Read the model definition and answer for the solid it produces. Units are mm, in the model's axes. A direction names the side the tool comes from. Give positions to 0.01 mm unless a question says otherwise; leave off trailing zeros. Write each loop counter-clockwise with the first axis right and the second up, starting at its lowest first coordinate (ties: lowest second). Pieces come first, ordered by that corner, then holes.
```python
from build123d import *

# Parameters (mm, degrees)
F0_W     = 7.8
F0_H     = 7.8
F1_DEPTH = 1
F2_SIZE2 = 0.5
F2_SIZE  = 7.8


# Not quite as in the source:
# - a feature names something its author has since deleted; it is built from what else it names


with BuildPart() as f1:
    # F0 (on Right) → F1 (new body)
    with BuildSketch(Plane.YZ):
        with BuildLine():
            Line((-3.9, 1.419822283), (3.9, 1.419822283))
            Line((3.9, 1.419822283), (4.5596052461, 1.419822283))
            ThreePointArc((4.5596052461, 1.419822283), (0, 3.519822283), (-4.5596052461, 1.419822283))
            Line((-4.5596052461, 1.419822283), (-3.9, 1.419822283))
        make_face()
        with Locations((0, -2.480177717)):
            Rectangle(F0_W, F0_H)
    extrude(amount=F1_DEPTH)

    # F2
    f2_edges = [f1.edges().sort_by_distance(p)[0] for p in [
        (0, 0, -6.380178),
    ]]
    f2_side = f1.faces().sort_by_distance((0, 0, -1.62771))[0]
    chamfer(f2_edges, length=F2_SIZE, length2=F2_SIZE2, reference=f2_side)


solid = f1.part
```
Item 1: Section D-D (y = -0.25) is taken. Write down the section's boundary in (x, z), and give its area (3 significant figures).
Result set:
outline: (0, 1.42) - (0.5, -6.38) - (1, -6.38) - (1, 3.51) - (0, 3.51) - close
area: 7.94 mm2
Item 2: Section C-C (z = -0.25) is taken. Write down the section's boundary in (x, y), and give its area (3 significant figures).
Result set:
outline: (0.11, -3.9) - (1, -3.9) - (1, 3.9) - (0.11, 3.9) - close
area: 6.97 mm2
Item 3: Which of the six approach directions +Z, -Z, +X, -X, +Y, -Y give full straight-line access (tool end or side, diameter ignored) to faces 1 (the flat face through (0.6, -3.9, -2.5)), 2 (the flat face through (0.6, 3.9, -2.5)), 3 (the cylindrical face through (0.49, 0.07, 3.52))?
Result set:
face 1: -Z, +X, -X, -Y
face 2: -Z, +X, -X, +Y
face 3: +Z, +X, -X
Item 4: Section B-B (y = -3.75) is taken. Write down the section's boundary in (x, z).
Result set:
outline: (0, 1.42) - (0.5, -6.38) - (1, -6.38) - (1, 2.2) - (0, 2.2) - close
Item 5: Section A-A (x = 0.7) is taken. Write down the section's boundary in (y, z).
Result set:
outline: (-4.56, 1.42) - (-3.9, 1.42) - (-3.9, -6.38) - (3.9, -6.38) - (3.9, 1.42) - (4.56, 1.42) arc R6 ccw to start
Item 6: This flat-tipped pin is pushed along its axis until it touches: pin 1 Ø4 at (y, z) = (-1.5, -1) entering from -X. Where does it stop, or does it pass through?
Result set:
pin 1: stops at x = 0.03
Item 7: Find the intervals of material crossed by line 1 along Y through (x, z) = (0.9, -1.75); line 2 along X through (y, z) = (0.25, -6); line 3 along Z through (x, y) = (0.9, 4.25), in increasing order.
Result set:
line 1: y = -3.9 to 3.9
line 2: x = 0.48 to 1
line 3: z = 1.42 to 1.76
